```python
from build123d import *

# Parameters (mm, degrees)
BOSS_EXTRUDE1_DEPTH     = 10
SKETCH2_R               = 17.5
CUT_EXTRUDE1_DEPTH      = 569.981596971
CUT_EXTRUDE2_DEPTH      = 562.341005262
CUT_EXTRUDE2_DEPTH_BACK = 562.341005262
SKETCH3_R               = 252.5


with BuildPart() as part:
    # Sweep1: sweep along a curve in space
    with BuildLine() as sweep1_path:
        ThreePointArc((0, 120.083798472, 63.431105038), (0, -235.570766963, -163.145841721), (0, 120.083798472, -389.72278848))
    # 3DSketch2 → Sweep1 (sweep)
    with BuildSketch(Plane(origin=(125, 120.083798472, 78.431105038), x_dir=(-0.9928768384869221, 0, -0.11914522061843064), z_dir=(0, -1, 0))):
        Polygon((0, 0), (3.574356619, 29.786305155), (251.79356624, 0), (248.219209622, -29.786305155), align=None)
    sweep(path=sweep1_path.line)

    # Sketch1 → Boss-Extrude1 (add, symmetric)
    with BuildSketch(Plane.XY):
        with BuildLine():
            Line((-67.5, -275), (-67.5, -175))
            Line((-67.5, -175), (67.5, -175))
            Line((67.5, -175), (67.5, -275))
            ThreePointArc((67.5, -275), (0, -342.5), (-67.5, -275))
        make_face()
    boss_extrude1 = extrude(amount=BOSS_EXTRUDE1_DEPTH, both=True)

    # Sketch2 → Cut-Extrude1 (cut, through all)
    with BuildSketch(Plane.XY.offset(10)):
        with Locations((0, -275)):
            Circle(SKETCH2_R)
    cut_extrude1 = extrude(amount=-CUT_EXTRUDE1_DEPTH, mode=Mode.SUBTRACT)

    # Mirror1: Boss-Extrude1, Cut-Extrude1 across plane
    add(boss_extrude1.mirror(Plane(origin=(0, 0, -157.91266462), x_dir=(1, 0, 0), z_dir=(0, 0, -1))))
    add(cut_extrude1.mirror(Plane(origin=(0, 0, -157.91266462), x_dir=(1, 0, 0), z_dir=(0, 0, -1))), mode=Mode.SUBTRACT)

    # Sketch3 → Cut-Extrude2 (cut, two sides: drawn at the far end of the back side and taken through both)
    with BuildSketch(Plane(origin=(0, 0, 0), x_dir=(0, 0, -1), z_dir=(1, 0, 0)).offset(-CUT_EXTRUDE2_DEPTH_BACK)):
        with Locations((163.145841721, 14.429233037)):
            Circle(SKETCH3_R)
    extrude(amount=CUT_EXTRUDE2_DEPTH + CUT_EXTRUDE2_DEPTH_BACK, mode=Mode.SUBTRACT)


solid = part.part
```
Could you check a few things on this model? Use its own coordinates, in mm. A direction names the side the tool comes from. Coordinates: 2 decimals unless noted, no trailing zeros. Order: outer loops, then holes, each group sorted by start corner. A loop starts at its lowest first (then second) coordinate and runs counter-clockwise, first axis right, second up. Notation, with made-up numbers: M -13,-9 L 6,-9 A35 ccw 6,25 Z; hole C 9,40 d7. An arc over 180 degrees is marked long. Use one line per item in the form item = value. Start each with the question number.
1. Suppose I cut it at C-C on z = -2.5. Write out the boundary of the cut face in (x, y).
2. For pin 1 (5 mm diameter, centred on x = -59.5, y = -101.5, fed in from +Z); pin 2 (1.5 mm diameter, centred on x = 85.5, y = -194.5, fed in from -Z); pin 3 (10 mm diameter, centred on x = -5, z = 71, fed in from +Y), each with a flat end and sliding along its axis, tell me the tip position at first contact or that it passes through.
3. On a 3-axis mill with a long thin cutter (end or side, diameter ignored), from which of +Z, -Z, +X, -X, +Y, -Y can I reach the whole of each face in a straight line? I mean faces 1 (the flat face through (1, -255, -10)), 2 (the flat face through (1, -250, -325.825)), 3 (the flat face through (-67.5, -230, 0)), 4 (the flat face through (67.5, -233, -316)), 5 (the flat face through (1, -245, 10)). Say none if no direction works.
4. Suppose I cut it at B-B on y = 2.5. Write out the boundary of the cut face in (x, z) (3 decimals).
5. Suppose I cut it at D-D on x = 49. Write out the boundary of the cut face in (y, z).
6. Please list where these lines run through material, in increasing order: line 1 (Z direction, x = 8, y = -304); line 2 (Z direction, x = 5.5, y = -53); line 3 (Y direction, x = 0, z = -320).
7. Suppose I cut it at A-A on x = 0. Write out the boundary of the cut face in (y, z), then the cut area to 3 significant figures.
8. We'd pull the mould along Y, two halves only. Please class faces 6 (the cylindrical face through (-1.8, -238, -157.2)), 7 (the flat face through (67.5, -229, 0)), 8 (the cylindrical face through (1.484, -342.484, 0.14)), 9 (the flat face through (2, 120.084, 72)): +Y half, -Y half, draft (parallel to the pull), parting line (faces both ways), or undercut.
Geometry says:
q1.outline = M -125,-194.65 L -67.5,-194.65 L -67.5,-275 A67.5 ccw 67.5,-275 L 67.5,-194.65 L 125,-194.65 L 125,-180.38 L -125,-180.38 Z; hole C 0,-275 d35
q2.pin_1 = 74.88
q2.pin_2 = -324.96
q2.pin_3 = 120.08
q3.face_1 = +X, -X, -Y
q3.face_2 = -Z, +X, -X, -Y
q3.face_3 = +Z, -X, -Y
q3.face_4 = -Z, +X, -Y
q3.face_5 = +Z, +X, -X, -Y
q4.outline = M -125,-426.547 L 125,-426.547 L 125,-415.364 L -125,-415.364 Z; M -125,89.072 L 125,89.072 L 125,100.255 L -125,100.255 Z
q5.outline = M -321.42,-325.83 L -193.07,-325.83 A263.67 ccw 131.57,-399.36 L 122.19,-391.49 A252.5 cw long 120.08,66.19 L 120.08,78.43 A263.67 ccw -184.42,10 L -321.42,10 L -321.42,-10 L -200.21,-10 A263.67 ccw -207.3,-305.83 L -321.42,-305.83 Z
q6.line_1 = -325.83 to -305.83, -10 to 10
q6.line_2 = -418.05 to -406.48, 80.18 to 91.76
q6.line_3 = -342.5 to -292.5, -257.5 to -183.44
q7.outline = M -342.5,-325.83 L -292.5,-325.83 L -292.5,-305.83 L -342.5,-305.83 Z; M -342.5,-10 L -292.5,-10 L -292.5,10 L -342.5,10 Z; M -257.5,-325.83 L -193.07,-325.83 A263.67 ccw 131.57,-399.36 L 122.19,-391.49 A252.5 cw long 120.08,66.19 L 120.08,78.43 A263.67 ccw -184.42,10 L -257.5,10 L -257.5,-10 L -200.21,-10 A263.67 ccw -207.3,-305.83 L -257.5,-305.83 Z
q7.area = 16,000 mm^2
q8.face_6 = undercut
q8.face_7 = draft
q8.face_8 = -Y half
q8.face_9 = +Y half
